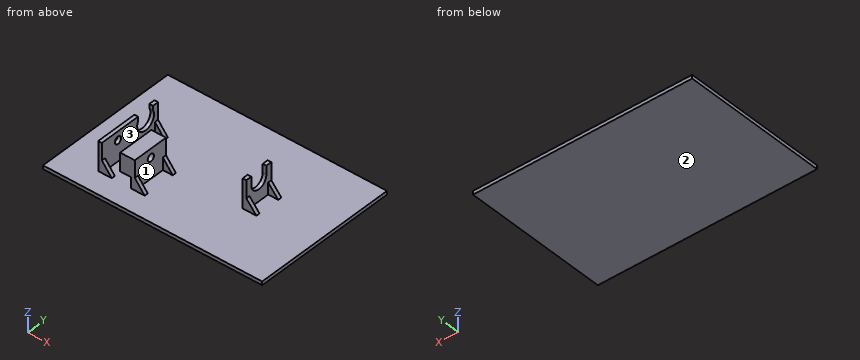
from build123d import *

# Parameters (mm, degrees)
SKETCH1_W            = 300
SKETCH1_H            = 200
BOSS_EXTRUDE1_DEPTH  = 5
SKETCH3_W            = 20
SKETCH3_H            = 20
SKETCH3_H_2          = 40
CUT_EXTRUDE1_DEPTH   = 5
SKETCH4_W            = 20
SKETCH4_H            = 40
CUT_EXTRUDE2_DEPTH   = 10
SKETCH6_W            = 300
SKETCH6_H            = 200
BOSS_EXTRUDE2_DEPTH  = 5
BOSS_EXTRUDE4_DEPTH  = 40
SKETCH8_3_W          = 5
SKETCH8_3_H          = 40
BOSS_EXTRUDE5_DEPTH  = 40
CUT_EXTRUDE3_DEPTH   = 236
SKETCH10_R           = 5
CUT_EXTRUDE4_DEPTH   = 236
BOSS_EXTRUDE6_DEPTH  = 5
BOSS_EXTRUDE7_DEPTH  = 5
BOSS_EXTRUDE8_DEPTH  = 5
CUT_EXTRUDE5_DEPTH   = 10
SKETCH19_W           = 25
SKETCH19_H           = 50
BOSS_EXTRUDE10_DEPTH = 15
BOSS_EXTRUDE11_DEPTH = 5
SKETCH22_R           = 5
CUT_EXTRUDE6_DEPTH   = 39
SKETCH23_R           = 13.5
CUT_EXTRUDE7_DEPTH   = 10


with BuildPart() as part:
    # Sketch1 → Boss-Extrude1 (new body)
    with BuildSketch(Plane.XY):
        Rectangle(SKETCH1_W, SKETCH1_H)
    extrude(amount=BOSS_EXTRUDE1_DEPTH)

    # Sketch3 → Cut-Extrude1 (cut)
    with BuildSketch(Plane.XY.offset(5)):
        with Locations((-140, -90)):
            Rectangle(SKETCH3_W, SKETCH3_H)
        with Locations((-140, 80)):
            Rectangle(SKETCH3_W, SKETCH3_H_2)
        with Locations((140, 80)):
            Rectangle(SKETCH3_W, SKETCH3_H_2)
        with Locations((140, -90)):
            Rectangle(SKETCH3_W, SKETCH3_H)
    extrude(amount=-CUT_EXTRUDE1_DEPTH, mode=Mode.SUBTRACT)

    # Sketch4 → Cut-Extrude2 (cut)
    with BuildSketch(Plane(origin=(0, 0, 0), x_dir=(-1, 0, 0), z_dir=(0, 0, -1))):
        with Locations((-140, -80)):
            Rectangle(SKETCH4_W, SKETCH4_H)
        with Locations((140, -80)):
            Rectangle(SKETCH4_W, SKETCH4_H)
    extrude(amount=-CUT_EXTRUDE2_DEPTH, mode=Mode.SUBTRACT)

    # Sketch6 → Boss-Extrude2 (add)
    with BuildSketch(Plane(origin=(0, 0, 0), x_dir=(-1, 0, 0), z_dir=(0, 0, -1))):
        Rectangle(SKETCH6_W, SKETCH6_H)
    extrude(amount=-BOSS_EXTRUDE2_DEPTH)

    # Sketch8 → Boss-Extrude4 (add)
    with BuildSketch(Plane.XY.offset(5)):
        Polygon((-100, 20), (-95, 20), (-95, -20), (-95, -70), (-100, -70), (-100, -20), align=None)
    boss_extrude4 = extrude(amount=BOSS_EXTRUDE4_DEPTH)

    # Sketch8<3> → Boss-Extrude5 (add)
    with BuildSketch(Plane.XY.offset(5)):
        with Locations((57.5, 0)):
            Rectangle(SKETCH8_3_W, SKETCH8_3_H)
    extrude(amount=BOSS_EXTRUDE5_DEPTH)

    # Sketch9 → Cut-Extrude3 (cut)
    with BuildSketch(Plane(origin=(60, 0, 0), x_dir=(0, 0, -1), z_dir=(1, 0, 0))):
        with BuildLine():
            Line((-45, 12), (-33, 12))
            ThreePointArc((-33, 12), (-21, 0), (-33, -12))
            Line((-33, -12), (-45, -12))
            Line((-45, -12), (-45, 12))
        make_face()
    extrude(amount=-CUT_EXTRUDE3_DEPTH, mode=Mode.SUBTRACT)

    # Sketch10 → Cut-Extrude4 (cut)
    with BuildSketch(Plane(origin=(-95, 0, 0), x_dir=(0, 0, -1), z_dir=(1, 0, 0))):
        with Locations((-33, -44.279864558)):
            Circle(SKETCH10_R)
    cut_extrude4 = extrude(amount=-CUT_EXTRUDE4_DEPTH, mode=Mode.SUBTRACT)

    # Sketch11 → Boss-Extrude6 (add)
    with BuildSketch(Plane.XZ.offset(70)):
        Polygon((-95, 21.66038922), (-81.566809401, 5), (-95, 5), align=None)
    extrude(amount=-BOSS_EXTRUDE6_DEPTH)

    # Sketch12 → Boss-Extrude7 (add)
    with BuildSketch(Plane(origin=(0, 20, 0), x_dir=(1, 0, 0), z_dir=(0, 1, 0))):
        Polygon((60, -21), (73.767048753, -5), (60, -5), align=None)
    boss_extrude7 = extrude(amount=-BOSS_EXTRUDE7_DEPTH)

    # Sketch12<3> → Boss-Extrude8 (add)
    with BuildSketch(Plane(origin=(0, 20, 0), x_dir=(1, 0, 0), z_dir=(0, 1, 0))):
        Polygon((-81.566809401, -5), (-95, -21.66038922), (-95, -5), align=None)
    extrude(amount=-BOSS_EXTRUDE8_DEPTH)

    # Mirror1: Boss-Extrude7 across plane
    add(boss_extrude7.mirror(Plane(origin=(0, 0, 0), x_dir=(0, 0, 1), z_dir=(0, -1, 0))))

    # Mirror3: Boss-Extrude4, Cut-Extrude4 across plane
    add(boss_extrude4.mirror(Plane(origin=(-75, 0, 0), x_dir=(0, 0, 1), z_dir=(1, 0, 0))))
    add(cut_extrude4.mirror(Plane(origin=(-75, 0, 0), x_dir=(0, 0, 1), z_dir=(1, 0, 0))), mode=Mode.SUBTRACT)

    # Sketch17 → Cut-Extrude5 (cut)
    with BuildSketch(Plane.ZY.offset(55)):
        Polygon((5, -20), (45, -20), (45, -12), (45, 20), (5, 20), align=None)
    extrude(amount=-CUT_EXTRUDE5_DEPTH, mode=Mode.SUBTRACT)

    # Sketch19 → Boss-Extrude10 (add)
    with BuildSketch(Plane.ZY.offset(55)):
        with Locations((32.5, -45)):
            Rectangle(SKETCH19_W, SKETCH19_H)
    extrude(amount=BOSS_EXTRUDE10_DEPTH)

    # Sketch20 → Boss-Extrude11 (add)
    with BuildSketch(Plane.XZ.offset(70)):
        Polygon((-50, 21.717977163), (-36.483235136, 5), (-50, 5), align=None)
    boss_extrude11 = extrude(amount=-BOSS_EXTRUDE11_DEPTH)

    # Mirror4: Boss-Extrude11 across plane
    add(boss_extrude11.mirror(Plane.ZX.offset(-45)))

    # Sketch22 → Cut-Extrude6 (cut)
    with BuildSketch(Plane(origin=(-75, 0, 0), x_dir=(0, 0, -1), z_dir=(1, 0, 0))):
        with Locations((-33, -44.279864558)):
            Circle(SKETCH22_R)
    extrude(amount=CUT_EXTRUDE6_DEPTH, mode=Mode.SUBTRACT)

    # Sketch23 → Cut-Extrude7 (cut)
    with BuildSketch(Plane.ZY.offset(100)):
        with Locations((33, 0)):
            Circle(SKETCH23_R)
    extrude(amount=-CUT_EXTRUDE7_DEPTH, mode=Mode.SUBTRACT)


solid = part.part
CAD build for the part. Positions are in the model's coordinates, mm. Face numbers are marked on the shaded views. Round coordinates to 2 decimals unless told otherwise and drop trailing zeros. Write each loop counter-clockwise with the first axis right and the second up, starting at its lowest first coordinate (ties: lowest second). Pieces come first, ordered by that corner, then holes.
(1) Slice it at C-C, the plane x = 28. Write the cut outline in (y, z).
(2) Probe line 1 along Y through (x, z) = (-98.25, 33); line 2 along X through (y, z) = (-64, 38); line 3 along X through (y, z) = (-27.5, 10.5). List the from-to ranges inside material, lowest first.
(3) Slice it at A-A, the plane z = 9. Write the cut outline in (x, y).
(4) Mould opens along X. For the marked faces 1, 2 and 3 say: pulls with the +X half, pulls with the -X half, needs draft (parallel to the pull), parting line crosses it, or undercut.
(5) Slice it at D-D, the plane y = 70. Write the cut outline in (x, z).
(6) Slice it at B-B, the plane y = 0. Write the cut outline in (x, z), and give its area (3 significant figures).
(7) Drop flat-ended pins along their axis: P1, Ø11.5, axis at y = -44.28, z = 33, coming from the +X side; P2, Ø20.5, axis at x = 67, z = 23.5, coming from the -Y side; P3, Ø15, axis at x = 62, z = 29, coming from the +Y side. Give the stop position or say it passes through.
From the geometry:
1. outline: (-100, 0) - (100, 0) - (100, 5) - (-100, 5) - close
2. line 1: y = -70 to -49.28, -39.28 to -13.5, 13.5 to 20
2. line 2: x = -100 to -95, -70 to -50
2. line 3: x = -100 to -95, -55 to -50
3. outline: (-100, -70) - (-84.79, -70) - (-84.79, -65) - (-95, -65) - (-95, 15) - (-84.79, 15) - (-84.79, 20) - (-100, 20) - close; (-55, -70) - (-39.72, -70) - (-39.72, -65) - (-50, -65) - (-50, -25) - (-39.72, -25) - (-39.72, -20) - (-55, -20) - close; (55, -20) - (70.33, -20) - (70.33, -15) - (60, -15) - (60, 15) - (70.33, 15) - (70.33, 20) - (55, 20) - close
4. face 1: pulls with the +X half
4. face 2: needs draft
4. face 3: undercut
5. outline: (-150, 0) - (150, 0) - (150, 5) - (-150, 5) - close
6. outline: (-150, 0) - (150, 0) - (150, 5) - (60, 5) - (60, 21) - (55, 21) - (55, 5) - (-95, 5) - (-95, 19.5) - (-100, 19.5) - (-100, 5) - (-150, 5) - close
6. area: 1,650 mm2
7. P1: stops at x = -50
7. P2: stops at y = -20
7. P3: stops at y = 20
